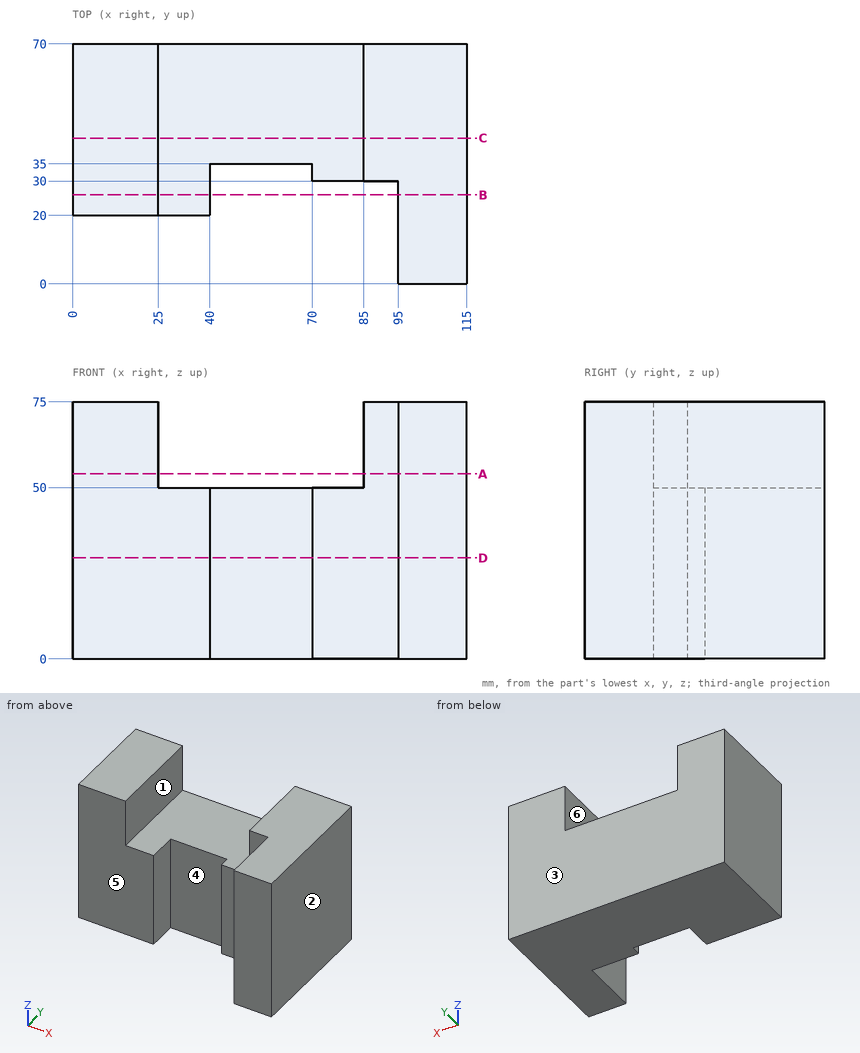
Geometry check sheet. Reference: drawing and pictorial views, mm from the part's lowest x, y, z. A direction names the side the tool comes from. Coordinates: 2 decimals unless noted, no trailing zeros. Order: outer loops, then holes, each group sorted by start corner. A loop starts at its lowest first (then second) coordinate and runs counter-clockwise, first axis right, second up. Notation, with made-up numbers: M -24,1 L 21,1 A25 ccw 21,23 Z; hole C 89,53.25 d6. An arc over 180 degrees is marked long. Return JSON: item names as keys, results as strings.
1) Cross-section at B-B, the plane y = 26. Record the boundary of the cut face in (x, z), and give its area (4 significant figures).
Answer list:
{"outline": "M 0,0 L 40,0 L 40,50 L 25,50 L 25,75 L 0,75 Z; M 95,0 L 115,0 L 115,75 L 95,75 Z", "area": "4,125 mm2"}
2) Access from +Z, -Z, +X, -X, +Y, -Y to the whole of each face (thin tool, end or side, straight path). Record for the marked faces 4, 5 and 6.
Answer list:
{"face 4": "+Z, -Z, -Y", "face 5": "+Z, -Z, -X, -Y", "face 6": "+Z, +Y, -Y"}
3) Cross-section at D-D, the plane z = 29.5. Record the boundary of the cut face in (x, y).
Answer list:
{"outline": "M 0,20 L 40,20 L 40,35 L 70,35 L 70,30 L 95,30 L 95,0 L 115,0 L 115,70 L 0,70 Z"}
4) Cross-section at A-A, the plane z = 54. Record the boundary of the cut face in (x, y).
Answer list:
{"outline": "M 0,20 L 25,20 L 25,70 L 0,70 Z; M 85,30 L 95,30 L 95,0 L 115,0 L 115,70 L 85,70 Z"}
5) Cross-section at C-C, the plane y = 42.5. Record the boundary of the cut face in (x, z), and give its area (4 significant figures).
Answer list:
{"outline": "M 0,0 L 115,0 L 115,75 L 85,75 L 85,50 L 25,50 L 25,75 L 0,75 Z", "area": "7,125 mm2"}
6) Thickness scan on L1, parallel to X at y = 40, z = 52; L2, parallel to X at y = 31, z = 36.5; L3, parallel to Y at x = 43.5, z = 41. Record the ranges inside material, lowest first. Write a range as [from, to].
Answer list:
{"L1": "[0, 25], [85, 115]", "L2": "[0, 40], [70, 115]", "L3": "[35, 70]"}
7) Gauge pin test, flat ends, axial feed: pin 1 (5.5 mm diameter, centred on y = 32, z = 30.5, fed in from -X); pin 2 (2 mm diameter, centred on x = 19.5, z = 45, fed in from -Y); pin 3 (1 mm diameter, centred on x = 75.5, z = 49.5, fed in from -Y); pin 4 (15 mm diameter, centred on x = 48.5, z = 34, fed in from -Y). Record the tip position at first contact, or that the pin passes through.
Answer list:
{"pin 1": "x = 0", "pin 2": "y = 20", "pin 3": "y = 30", "pin 4": "y = 35"}
8) Release check for a two-part mould opening along X. For the marked faces 1, 2 and 3 record: +X half, -X half, draft (parallel to the pull), parting line (faces both ways), or undercut.
Answer list:
{"face 1": "undercut", "face 2": "+X half", "face 3": "draft"}
